CAD build for the part. Positions are in the model's coordinates, mm. Face numbers are marked on the shaded views. A direction names the side the tool comes from. Coordinates: 2 decimals unless noted, no trailing zeros. Loops run counter-clockwise (first coordinate to the right, second up) from the corner with the lowest first, then second, coordinate; pieces in that order, holes last. Notation, with made-up numbers: (78, -12) -> (137, -12) arc R20 cw to (137, 9) -> close; hole circle Ø4 at (-37, 80.5). An arc over 180 degrees is marked (long way). Write each question's results on one line, items separated by ' | '.
from build123d import *

# Parameters (mm, degrees)
SKETCH1_W                = 46.5
SKETCH1_H                = 35.6
BOSS_EXTRUDE1_DEPTH      = 2
SKETCH2_W                = 3
SKETCH2_H                = 35.6
BOSS_EXTRUDE2_DEPTH      = 50
SKETCH3_R                = 4.25
CUT_EXTRUDE1_DEPTH       = 47.5
SKETCH6_R                = 1.25
CUT_EXTRUDE3_DEPTH       = 47.5
FILLET5_R                = 16
SKETCH1_2_W              = 46.5
SKETCH1_2_H              = 35.6
CUT_EXTRUDE6_DEPTH       = 20
SKETCH8_W                = 46.5
SKETCH8_H                = 35.6
BOSS_EXTRUDE3_DEPTH      = 3
SKETCH9_W                = 35.6
SKETCH9_H                = 13
BOSS_EXTRUDE4_DEPTH      = 46.5
SKETCH12_W               = 30
SKETCH12_H               = 13
CUT_EXTRUDE9_DEPTH       = 36.6
SKETCH13_W               = 24.4
SKETCH13_H               = 13
CUT_EXTRUDE10_DEPTH      = 39.25
CUT_EXTRUDE10_DEPTH_BACK = 9.25
SKETCH15_R               = 1.35
CUT_EXTRUDE11_DEPTH      = 47.5


with BuildPart() as part:
    # Sketch1 → Boss-Extrude1 (new body)
    with BuildSketch(Plane(origin=(0, 0, 0), x_dir=(1, 0, 0), z_dir=(0, 1, 0))):
        Rectangle(SKETCH1_W, SKETCH1_H)
    extrude(amount=BOSS_EXTRUDE1_DEPTH)

    # Sketch2 → Boss-Extrude2 (add)
    with BuildSketch(Plane(origin=(0, 2, 0), x_dir=(1, 0, 0), z_dir=(0, 1, 0))):
        with Locations((-21.75, 0)):
            Rectangle(SKETCH2_W, SKETCH2_H)
        with Locations((21.75, 0)):
            Rectangle(SKETCH2_W, SKETCH2_H)
    extrude(amount=BOSS_EXTRUDE2_DEPTH)

    # Sketch3 → Cut-Extrude1 (cut, through all)
    with BuildSketch(Plane(origin=(23.25, 0, 0), x_dir=(0, 0, -1), z_dir=(1, 0, 0))):
        with Locations((0, 40)):
            Circle(SKETCH3_R)
    extrude(amount=-CUT_EXTRUDE1_DEPTH, mode=Mode.SUBTRACT)

    # Sketch6 → Cut-Extrude3 (cut, through all)
    with BuildSketch(Plane(origin=(23.25, 0, 0), x_dir=(0, 0, -1), z_dir=(1, 0, 0))):
        with Locations((0, 32)):
            Circle(SKETCH6_R)
        with Locations((-5.656854249, 34.343145751)):
            Circle(SKETCH6_R)
        with Locations((-8, 40)):
            Circle(SKETCH6_R)
        with Locations((-5.656854249, 45.656854249)):
            Circle(SKETCH6_R)
        with Locations((0, 48)):
            Circle(SKETCH6_R)
        with Locations((5.656854249, 45.656854249)):
            Circle(SKETCH6_R)
        with Locations((8, 40)):
            Circle(SKETCH6_R)
        with Locations((5.656854249, 34.343145751)):
            Circle(SKETCH6_R)
    extrude(amount=-CUT_EXTRUDE3_DEPTH, mode=Mode.SUBTRACT)

    # Fillet5
    fillet5_edges = [part.edges().sort_by_distance(p)[0] for p in [
        (-21.75, 52, 17.8),
        (-21.75, 52, -17.8),
        (21.75, 52, -17.8),
        (21.75, 52, 17.8),
    ]]
    fillet(fillet5_edges, radius=FILLET5_R)

    # Sketch1<2> → Cut-Extrude6 (cut)
    with BuildSketch(Plane(origin=(0, 0, 0), x_dir=(1, 0, 0), z_dir=(0, 1, 0))):
        Rectangle(SKETCH1_2_W, SKETCH1_2_H)
    extrude(amount=CUT_EXTRUDE6_DEPTH, mode=Mode.SUBTRACT)

    # Sketch8 → Boss-Extrude3 (add)
    with BuildSketch(Plane.XZ.offset(-20)):
        Rectangle(SKETCH8_W, SKETCH8_H)
    extrude(amount=BOSS_EXTRUDE3_DEPTH)

    # Sketch9 → Boss-Extrude4 (add)
    with BuildSketch(Plane(origin=(23.25, 0, 0), x_dir=(0, 0, -1), z_dir=(1, 0, 0))):
        with Locations((0, 10.5)):
            Rectangle(SKETCH9_W, SKETCH9_H)
    extrude(amount=-BOSS_EXTRUDE4_DEPTH)

    # Sketch12 → Cut-Extrude9 (cut, through all)
    with BuildSketch(Plane(origin=(0, 0, -17.8), x_dir=(-1, 0, 0), z_dir=(0, 0, -1))):
        with Locations((0, 10.5)):
            Rectangle(SKETCH12_W, SKETCH12_H)
    extrude(amount=-CUT_EXTRUDE9_DEPTH, mode=Mode.SUBTRACT)

    # Sketch13 → Cut-Extrude10 (cut, two sides)
    with BuildSketch(Plane.ZY.offset(-15)) as cut_extrude10_sk:
        with Locations((0, 10.5)):
            Rectangle(SKETCH13_W, SKETCH13_H)
    extrude(amount=CUT_EXTRUDE10_DEPTH, mode=Mode.SUBTRACT)
    extrude(cut_extrude10_sk.sketch, amount=-CUT_EXTRUDE10_DEPTH_BACK, mode=Mode.SUBTRACT)

    # Sketch15 → Cut-Extrude11 (cut, through all)
    with BuildSketch(Plane.ZY.offset(23.25)):
        with Locations((-15, 6.9)):
            Circle(SKETCH15_R)
        with Locations((15, 6.9)):
            Circle(SKETCH15_R)
    extrude(amount=-CUT_EXTRUDE11_DEPTH, mode=Mode.SUBTRACT)


solid = part.part
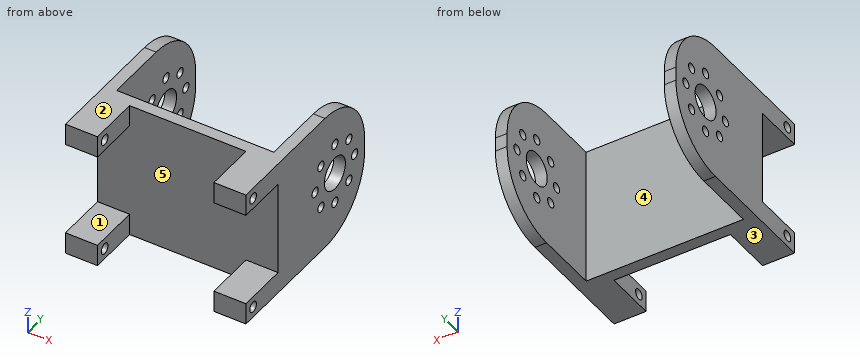
1) Slice it at B-B (x = -16). Write the cut outline in (y, z), then the cut area to 3 significant figures.
Outcome:
outline: (4, -17.8) -> (20, -17.8) -> (20, 17.8) -> (4, 17.8) -> (4, 12.2) -> (17, 12.2) -> (17, -12.2) -> (4, -12.2) -> close; hole circle Ø2.7 at (6.9, -15); hole circle Ø2.7 at (6.9, 15) | area: 241 mm^2
2) Slice it at C-C (z = 0). Count the separate pieces of the cut face and the enclosed holes in it, then the cut area to 4 significant figures.
Outcome:
separate pieces: 7 | enclosed holes: 0 | area: 250.5 mm^2
3) Drill centre lines: L1, parallel to Y at x = -21, z = 0; L2, parallel to X at y = 23.5, z = 16; L3, parallel to Y at x = -20, z = -15. Where is each one in solid material? Low to high. Write a range as from..to.
Outcome:
L1: y = 17..30.75, 33.25..35.75, 44.25..46.75, 49.25..52 | L2: x = -23.25..-20.25, 20.25..23.25 | L3: y = 4..5.55, 8.25..20
4) Pin check, flat tips, straight feed: pin 1 (1.5 mm diameter, centred on x = 9.5, z = -14, fed in from +Y); pin 2 (8 mm diameter, centred on x = 10.5, z = 8.5, fed in from -Y). Stop position of each tip, or through.
Outcome:
pin 1: stops at y = 20 | pin 2: stops at y = 17
5) Which spindle directions (+Z, -Z, +X, -X, +Y, -Y) get a long thin tool onto all of the face, cutting with end or side? Do the marked faces 1, 2, 3, 4 and 5. Say none if no direction does.
Outcome:
face 1: +X, -X, -Y | face 2: +Z, +X, -X, +Y, -Y | face 3: -Z, +X, -X, +Y, -Y | face 4: +Z, -Z, +Y | face 5: -Y
6) Slice it at A-A (y = 12.5). Write the cut outline in (x, z).
Outcome:
outline: (-23.25, -17.8) -> (-15, -17.8) -> (-15, -12.2) -> (-23.25, -12.2) -> close; (-23.25, 12.2) -> (-15, 12.2) -> (-15, 17.8) -> (-23.25, 17.8) -> close; (15, -17.8) -> (23.25, -17.8) -> (23.25, -12.2) -> (15, -12.2) -> close; (15, 12.2) -> (23.25, 12.2) -> (23.25, 17.8) -> (15, 17.8) -> close
7) Slice it at D-D (z = -8). Write the cut outline in (x, y).
Outcome:
outline: (-23.25, 17) -> (23.25, 17) -> (23.25, 38.75) -> (20.25, 38.75) -> (20.25, 20) -> (-20.25, 20) -> (-20.25, 38.75) -> (-23.25, 38.75) -> close; (-23.25, 41.25) -> (-20.25, 41.25) -> (-20.25, 50.75) -> (-23.25, 50.75) -> close; (20.25, 41.25) -> (23.25, 41.25) -> (23.25, 50.75) -> (20.25, 50.75) -> close
